Read the model definition and answer for the solid it produces. Units are mm, in the model's axes. Face numbers are marked on the shaded views. Give positions to 0.01 mm unless a question says otherwise; leave off trailing zeros. Write each loop counter-clockwise with the first axis right and the second up, starting at its lowest first coordinate (ties: lowest second). Pieces come first, ordered by that corner, then holes. Notation, with made-up numbers: (9, -7.75) -> (24, -7.75) arc R26 ccw to (24, 26.25) -> close; hole circle Ø3 at (54, 37). An arc over 180 degrees is marked (long way). Use a Markdown table: item, result.
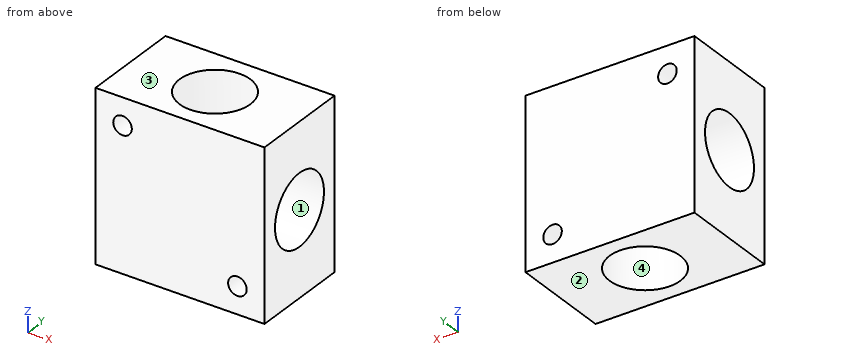
from build123d import *

# Parameters (mm, degrees)
F0_W     = 50
F0_H     = 50
F1_DEPTH = 30
F3_D     = 5.5
F4_R     = 10.48
F5_DEPTH = 50.001
F6_R     = 10.48
F7_DEPTH = 50.001


with BuildPart() as f1:
    # F0 (on Front) → F1 (new body)
    with BuildSketch(Plane.XZ):
        Rectangle(F0_W, F0_H)
    extrude(amount=F1_DEPTH)

    # F3 (through all)
    with Locations(Plane.XZ.offset(30)):
        with Locations((-17, 17), (17, -17)):
            Hole(F3_D / 2)

    # F4 (on face) → F5 (cut, through all)
    with BuildSketch(Plane.XY.offset(25)):
        with Locations((0, -15)):
            Circle(F4_R)
    extrude(amount=-F5_DEPTH, mode=Mode.SUBTRACT)

    # F6 (on face) → F7 (cut, through all)
    with BuildSketch(Plane(origin=(-25, 0, 0), x_dir=(0, -1, 0), z_dir=(-1, 0, 0))):
        with Locations((15, 0)):
            Circle(F6_R)
    extrude(amount=-F7_DEPTH, mode=Mode.SUBTRACT)


solid = f1.part
Item 1: A cutting plane is placed at B-B (y = -20). Give the vertices of the cut face in (x, z).
Return value:
| item | result |
|---|---|
| outline | (-25, -25) -> (-9.21, -25) -> (-9.21, -9.21) -> (-25, -9.21) -> close; (-25, 9.21) -> (-9.21, 9.21) -> (-9.21, 25) -> (-25, 25) -> close; (9.21, -25) -> (25, -25) -> (25, -9.21) -> (9.21, -9.21) -> close; (9.21, 9.21) -> (25, 9.21) -> (25, 25) -> (9.21, 25) -> close; hole circle Ø5.5 at (-17, 17); hole circle Ø5.5 at (17, -17) |
Item 2: Straight lines are drawn through the part: line 1 along X through (y, z) = (-15, 12); line 2 along Z through (x, y) = (-17, -11); line 3 along Z through (x, y) = (16, -21.5). For each, find the intervals that lie inside material, in ascending order. Write a range as [from, to].
Return value:
| item | result |
|---|---|
| line 1 | [-25, -10.48], [10.48, 25] |
| line 2 | [-25, -9.69], [9.69, 14.25], [19.75, 25] |
| line 3 | [-25, -19.56], [-14.44, -8.22], [8.22, 25] |
Item 3: A cutting plane is placed at C-C (x = 17). Give the vertices of the cut face in (y, z), then the cut area to 3 significant figures.
Return value:
| item | result |
|---|---|
| outline | (-30, -25) -> (0, -25) -> (0, -19.75) -> (-30, -19.75) -> close; (-30, -14.25) -> (0, -14.25) -> (0, 25) -> (-30, 25) -> close; hole circle Ø20.96 at (-15, 0) |
| area | 990 mm^2 |
Item 4: For a pull along Z with two mould halves and no side action, classify the marked faces 1, 2, 3 and 4 as +Z half, -Z half, draft (parallel to the pull), parting line (faces both ways), or undercut.
Return value:
| item | result |
|---|---|
| face 1 | undercut |
| face 2 | -Z half |
| face 3 | +Z half |
| face 4 | draft |
Item 5: This flat-tipped pin is pushed along its axis until it touches: P1, Ø12.5, axis at x = 0, y = -15, coming from the -Z side. Where does it stop, or does it pass through?
Return value:
| item | result |
|---|---|
| P1 | through |
Item 6: A cutting plane is placed at A-A (z = -17). Give the vertices of the cut face in (x, y), then the cut area to 3 significant figures.
Return value:
| item | result |
|---|---|
| outline | (-25, -30) -> (14.25, -30) -> (14.25, 0) -> (-25, 0) -> close; (19.75, -30) -> (25, -30) -> (25, 0) -> (19.75, 0) -> close; hole circle Ø20.96 at (0, -15) |
| area | 990 mm^2 |
Item 7: A cutting plane is placed at D-D (z = 21). Give the vertices of the cut face in (x, y), then the cut area to 3 significant figures.
Return value:
| item | result |
|---|---|
| outline | (-25, -30) -> (25, -30) -> (25, 0) -> (-25, 0) -> close; hole circle Ø20.96 at (0, -15) |
| area | 1,150 mm^2 |
